Could you check a few things on this model? Use its own coordinates, in mm. Face numbers are marked on the shaded views. Coordinates: 2 decimals unless noted, no trailing zeros. Loops run counter-clockwise (first coordinate to the right, second up) from the corner with the lowest first, then second, coordinate; pieces in that order, holes last.
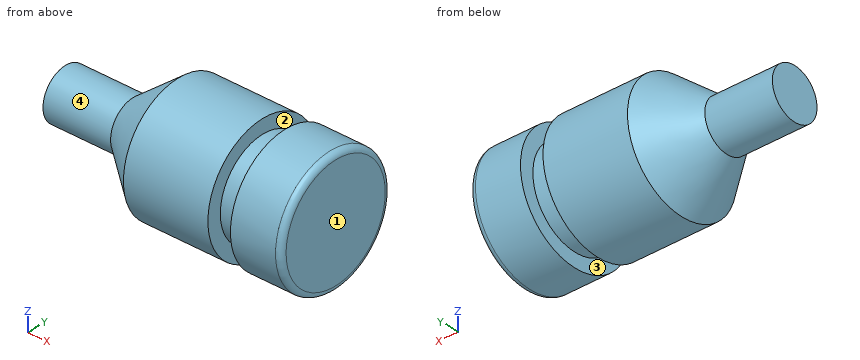
from build123d import *


with BuildPart() as f1:
    # F0 (on Front) → F1 (revolve)
    with BuildSketch(Plane.XZ):
        with BuildLine():
            Line((0, 22.5), (0, 0))
            Line((0, 0), (240, 0))
            Line((240, 0), (240, 50))
            ThreePointArc((240, 50), (238.535534, 53.535534), (235, 55))
            Line((235, 55), (195, 55))
            Line((195, 55), (195, 42.5))
            Line((195, 42.5), (175, 42.5))
            Line((175, 42.5), (175, 55))
            Line((175, 55), (100, 55))
            Line((100, 55), (60, 22.5))
            Line((60, 22.5), (0, 22.5))
        make_face()
    revolve(axis=Axis((-20.114416, 0, 0), (-1, 0, 0)))


solid = f1.part
(1) For pin 1 (2 mm diameter, centred on x = 36.5, y = 19, fed in from -Z); pin 2 (1.5 mm diameter, centred on x = 210.5, y = 28, fed in from -Z); pin 3 (1.5 mm diameter, centred on x = 88, y = -21.5, fed in from +Z), each with a flat end and sliding along its axis, tell me the tip position at first contact or that it passes through.
Answers:
pin 1: stops at z = -13.5
pin 2: stops at z = -47.77
pin 3: stops at z = 40.61
(2) Imagine slicing it at C-C, the plane x = 150. Write out the boundary of the cut face in (y, z).
Answers:
outline: circle Ø110 at (0, 0)
(3) Imagine slicing it at D-D, the plane x = 38.5. Write out the boundary of the cut face in (y, z).
Answers:
outline: circle Ø45 at (0, 0)
(4) We'd pull the mould along X, two halves only. Please class the marked faces 1, 2, 3 and 4: +X half, -X half, draft (parallel to the pull), parting line (faces both ways), or undercut.
Answers:
face 1: +X half
face 2: undercut
face 3: undercut
face 4: draft
(5) I need wall thicknesses on probe 1 along X at (y, z) = (-32, 28); probe 2 along X at (y, z) = (44.5, 30.5); probe 3 along Y at (x, z) = (197, 23). Which ranges of each line are inside material? Lowest first, please.
Answers:
probe 1: x = 84.64 to 175, 195 to 240
probe 2: x = 98.71 to 175, 195 to 238.07
probe 3: y = -49.96 to 49.96
(6) Imagine slicing it at A-A, the plane z = 0. Write out the boundary of the cut face in (x, y).
Answers:
outline: (0, -22.5) - (60, -22.5) - (100, -55) - (175, -55) - (175, -42.5) - (195, -42.5) - (195, -55) - (235, -55) arc R5 ccw to (240, -50) - (240, 50) arc R5 ccw to (235, 55) - (195, 55) - (195, 42.5) - (175, 42.5) - (175, 55) - (100, 55) - (60, 22.5) - (0, 22.5) - close
